Here's how the part is built. I have some questions about the finished solid (model axes, mm). A direction names the side the tool comes from. Coordinates: 2 decimals unless noted, no trailing zeros. Write each loop counter-clockwise with the first axis right and the second up, starting at its lowest first coordinate (ties: lowest second). Pieces come first, ordered by that corner, then holes. Notation, with made-up numbers: M 62.5,-26 L 75.5,-26 A13 cw 75.5,-1 Z; hole C 37.25,-2.75 d10. An arc over 180 degrees is marked long. Use a Markdown table: item, result.
```python
from build123d import *

# Parameters (mm, degrees)
F1_DEPTH     = 7.6
F2_R         = 1
F3_DEPTH     = 13.451
F4_R         = 3.8
F4_R_2       = 3.5
F4_R_3       = 2
F5_DEPTH     = 2
F6_DEPTH     = 2.17
F7_DEPTH     = 4.1
F8_T1_DEPTH  = 8.885841494
F8_T6_DEPTH  = 15.442920747
F8_S7_R      = 3.8
F8_T8_DEPTH  = 9
F8_T12_DEPTH = 15.442920747
F8_S13_R     = 3.8
F8_T14_DEPTH = 9
F8_T18_DEPTH = 4.442920747
F8_S19_R     = 3.8
F8_T20_DEPTH = 4
F8_T24_DEPTH = 4.442920747
F8_S25_R     = 3.8
F8_T26_DEPTH = 4
F8_T30_DEPTH = 4.442920747
F8_S31_R     = 3.8
F8_T32_DEPTH = 4
F8_T36_DEPTH = 4.442920747
F8_S37_R     = 3.8
F8_T38_DEPTH = 4


# Not quite as in the source:
# - a fillet or chamfer that OpenCascade refuses, or shapes differently, is made with other operations: its cross-section is extruded or revolved along the edge and cut away or added


with BuildPart() as f1:
    # F0 (on Front) → F1 (new body)
    with BuildSketch(Plane.XZ):
        Polygon((9.3, 15.7), (-9.3, 15.7), (-9.3, 13.45), (-13.3, 13.45), (-13.3, 11.95), (-9.3, 11.95), (-9.3, 0), (9.3, 0), (9.3, 11.95), (13.3, 11.95), (13.3, 13.45), (9.3, 13.45), align=None)
    extrude(amount=F1_DEPTH)

    # F2 (on face) → F3 (cut, through all)
    with BuildSketch(Plane.XY.offset(13.45)):
        with Locations((-11.3, -3.8)):
            Circle(F2_R)
        with Locations((11.3, -3.8)):
            Circle(F2_R)
    extrude(amount=-F3_DEPTH, mode=Mode.SUBTRACT)

    # F4 (on face) → F5 (join)
    with BuildSketch(Plane.XY.offset(15.7)):
        with Locations((5.5, -3.8)):
            Circle(F4_R)
        with Locations((5.5, -3.8)):
            Circle(F4_R_2, mode=Mode.SUBTRACT)
        with Locations((5.5, -3.8)):
            Circle(F4_R_2)
        with Locations((5.5, -3.8)):
            Circle(F4_R_3, mode=Mode.SUBTRACT)
        with Locations((5.5, -3.8)):
            Circle(F4_R_3)
    extrude(amount=F5_DEPTH)

    # F4 (on face) → F6 (join)
    with BuildSketch(Plane.XY.offset(15.7)):
        with Locations((5.5, -3.8)):
            Circle(F4_R_2)
        with Locations((5.5, -3.8)):
            Circle(F4_R_3, mode=Mode.SUBTRACT)
        with Locations((5.5, -3.8)):
            Circle(F4_R_3)
    extrude(amount=F6_DEPTH)

    # F4 (on face) → F7 (join)
    with BuildSketch(Plane.XY.offset(15.7)):
        with Locations((5.5, -3.8)):
            Circle(F4_R_3)
    extrude(amount=F7_DEPTH)

    # F8: chamfer of 0.25 on 7 edges, made by hand

    # F8_s2 → F8_t1 (cut)
    with BuildSketch(Plane.XZ.offset(-0.642920747)):
        Polygon((-9.05, 15.7), (-9.3, 15.45), (-9.3, 15.7), align=None)
    extrude(amount=F8_T1_DEPTH, mode=Mode.SUBTRACT)


with BuildPart() as f8_tool4:
    # F8_s5 → F8_t6 (new body)
    with BuildSketch(Plane.YZ.offset(5.5)):
        Polygon((-7.35, 15.7), (-7.6, 15.45), (-7.6, 15.7), align=None)
    extrude(amount=-F8_T6_DEPTH)

    # F8_s7 → F8_t8 (cut, symmetric)
    with BuildSketch(Plane.XY.offset(15.6)):
        with Locations((5.5, -3.8)):
            Circle(F8_S7_R)
    extrude(amount=F8_T8_DEPTH, both=True, mode=Mode.SUBTRACT)


with BuildPart() as f1_1:
    add(f1.part)

    # F8_t3: cut F8_tool4
    add(f8_tool4.part, mode=Mode.SUBTRACT)


with BuildPart() as f8_tool10:
    # F8_s11 → F8_t12 (new body)
    with BuildSketch(Plane.YZ.offset(5.5)):
        Polygon((0, 15.45), (-0.25, 15.7), (0, 15.7), align=None)
    extrude(amount=-F8_T12_DEPTH)

    # F8_s13 → F8_t14 (cut, symmetric)
    with BuildSketch(Plane.XY.offset(15.6)):
        with Locations((5.5, -3.8)):
            Circle(F8_S13_R)
    extrude(amount=F8_T14_DEPTH, both=True, mode=Mode.SUBTRACT)


with BuildPart() as f1_2:
    add(f1_1.part)

    # F8_t9: cut F8_tool10
    add(f8_tool10.part, mode=Mode.SUBTRACT)


with BuildPart() as f8_tool16:
    # F8_s17 → F8_t18 (new body)
    with BuildSketch(Plane.XZ.offset(3.8)):
        Polygon((9.3, 15.45), (9.05, 15.7), (9.3, 15.7), align=None)
    extrude(amount=F8_T18_DEPTH)

    # F8_s19 → F8_t20 (cut, symmetric)
    with BuildSketch(Plane.XY.offset(15.6)):
        with Locations((5.5, -3.8)):
            Circle(F8_S19_R)
    extrude(amount=F8_T20_DEPTH, both=True, mode=Mode.SUBTRACT)


with BuildPart() as f1_3:
    add(f1_2.part)

    # F8_t15: cut F8_tool16
    add(f8_tool16.part, mode=Mode.SUBTRACT)


with BuildPart() as f8_tool22:
    # F8_s23 → F8_t24 (new body)
    with BuildSketch(Plane.YZ.offset(9.942920747)):
        Polygon((-0.25, 15.7), (0, 15.45), (0, 15.7), align=None)
    extrude(amount=-F8_T24_DEPTH)

    # F8_s25 → F8_t26 (cut, symmetric)
    with BuildSketch(Plane.XY.offset(15.6)):
        with Locations((5.5, -3.8)):
            Circle(F8_S25_R)
    extrude(amount=F8_T26_DEPTH, both=True, mode=Mode.SUBTRACT)


with BuildPart() as f1_4:
    add(f1_3.part)

    # F8_t21: cut F8_tool22
    add(f8_tool22.part, mode=Mode.SUBTRACT)


with BuildPart() as f8_tool28:
    # F8_s29 → F8_t30 (new body)
    with BuildSketch(Plane.XZ.offset(-0.642920747)):
        Polygon((9.05, 15.7), (9.3, 15.45), (9.3, 15.7), align=None)
    extrude(amount=F8_T30_DEPTH)

    # F8_s31 → F8_t32 (cut, symmetric)
    with BuildSketch(Plane.XY.offset(15.6)):
        with Locations((5.5, -3.8)):
            Circle(F8_S31_R)
    extrude(amount=F8_T32_DEPTH, both=True, mode=Mode.SUBTRACT)


with BuildPart() as f1_5:
    add(f1_4.part)

    # F8_t27: cut F8_tool28
    add(f8_tool28.part, mode=Mode.SUBTRACT)


with BuildPart() as f8_tool34:
    # F8_s35 → F8_t36 (new body)
    with BuildSketch(Plane.YZ.offset(9.942920747)):
        Polygon((-7.35, 15.7), (-7.6, 15.45), (-7.6, 15.7), align=None)
    extrude(amount=-F8_T36_DEPTH)

    # F8_s37 → F8_t38 (cut, symmetric)
    with BuildSketch(Plane.XY.offset(15.6)):
        with Locations((5.5, -3.8)):
            Circle(F8_S37_R)
    extrude(amount=F8_T38_DEPTH, both=True, mode=Mode.SUBTRACT)


with BuildPart() as f1_6:
    add(f1_5.part)

    # F8_t33: cut F8_tool34
    add(f8_tool34.part, mode=Mode.SUBTRACT)


solid = f1_6.part
```
1. Suppose I cut it at A-A on x = 11.3. Write out the boundary of the cut face in (y, z).
Answers follow:
| item | result |
|---|---|
| outline | M -7.6,11.95 L -4.8,11.95 L -4.8,13.45 L -7.6,13.45 Z; M -2.8,11.95 L 0,11.95 L 0,13.45 L -2.8,13.45 Z |
2. Suppose I cut it at B-B on x = -0.5. Write out the boundary of the cut face in (y, z), and give its area (3 significant figures).
Answers follow:
| item | result |
|---|---|
| outline | M -7.6,0 L 0,0 L 0,15.45 L -0.25,15.7 L -7.35,15.7 L -7.6,15.45 Z |
| area | 119 mm2 |
3. Suppose I cut it at D-D on z = 18.25. Write out the boundary of the cut face in (x, y), and give its area (3 significant figures).
Answers follow:
| item | result |
|---|---|
| outline | C 5.5,-3.8 d4 |
| area | 12.6 mm2 |
4. Suppose I cut it at C-C on y = -1. Write out the boundary of the cut face in (x, z), and give its area (3 significant figures).
Answers follow:
| item | result |
|---|---|
| outline | M -13.3,11.95 L -9.3,11.95 L -9.3,0 L 9.3,0 L 9.3,11.95 L 13.3,11.95 L 13.3,13.45 L 9.3,13.45 L 9.3,15.45 L 9.05,15.7 L 8.07,15.7 L 8.07,17.7 L 7.6,17.7 L 7.6,17.87 L 3.4,17.87 L 3.4,17.7 L 2.93,17.7 L 2.93,15.7 L -9.05,15.7 L -9.3,15.45 L -9.3,13.45 L -13.3,13.45 Z |
| area | 315 mm2 |
5. Will these pins go through, and if not, where does the flat tip stop? pin 1 Ø2.5 at (x, y) = (8, -1.5) entering from +Z; pin 2 Ø3.5 at (x, y) = (-1, -5) entering from +Z; pin 3 Ø3 at (x, y) = (10.5, -2.5) entering from +Z.
Answers follow:
| item | result |
|---|---|
| pin 1 | stops at z = 17.87 |
| pin 2 | stops at z = 15.7 |
| pin 3 | stops at z = 17.7 |
6. Which directions (+Z, -Z, +X, -X, +Y, -Y) give clear straight access to the entire face, cutting with the end or side of a thin tool? Please do faces 1 (the face through (-10, -3, 13.45)), 2 (the face through (9.3, -4, 6)), 3 (the face through (4.026, -2.448, 18.821)).
Answers follow:
| item | result |
|---|---|
| face 1 | +Z, -X, +Y, -Y |
| face 2 | -Z, +X, +Y, -Y |
| face 3 | +Z |
7. I need wall thicknesses on probe 1 along Y at (x, z) = (11.3, 13.15); probe 2 along Z at (x, y) = (0.5, -1.75); probe 3 along X at (y, z) = (-3.75, 10). Which ranges of each line are inside material? Lowest first, please.
Answers follow:
| item | result |
|---|---|
| probe 1 | y = -7.6 to -4.8, -2.8 to 0 |
| probe 2 | z = 0 to 15.7 |
| probe 3 | x = -9.3 to 9.3 |
